Check sheet for the modelled part. Datum: model origin and axes. Units: mm. A direction names the side the tool comes from. Round coordinates to 2 decimals unless told otherwise and drop trailing zeros. Write each loop counter-clockwise with the first axis right and the second up, starting at its lowest first coordinate (ties: lowest second). Pieces come first, ordered by that corner, then holes. Notation, with made-up numbers: (-33.5, 33) -> (0.5, 33) arc R33 ccw to (0.5, 62) -> close; hole circle Ø7 at (8, -16.75). An arc over 180 degrees is marked (long way). One line per item, written item: value.
from build123d import *

# Parameters (mm, degrees)
SKETCH_1_R          = 3.9
SKETCH_1_R_2        = 2.2
SKETCH_1_R_3        = 1
EXTRUDE_1_DEPTH     = 0.8
SKETCH_1_4_R        = 2.2
SKETCH_1_4_R_2      = 1
EXTRUDE_2_DEPTH     = 3.2
FILLET_1_R          = 0.2
SKETCH_2_R          = 1.15
CUT_EXTRUDE_1_DEPTH = 0.5
CUT_EXTRUDE_2_REACH = 8.813


with BuildPart() as part:
    # Sketch 1 → Extrude 1 (new body)
    with BuildSketch(Plane.XY):
        Circle(SKETCH_1_R)
        Circle(SKETCH_1_R_2, mode=Mode.SUBTRACT)
        Circle(SKETCH_1_R_2)
        Circle(SKETCH_1_R_3, mode=Mode.SUBTRACT)
    extrude(amount=-EXTRUDE_1_DEPTH)

    # Sketch 1_4 → Extrude 2 (add)
    with BuildSketch(Plane.XY):
        Circle(SKETCH_1_4_R)
        Circle(SKETCH_1_4_R_2, mode=Mode.SUBTRACT)
    extrude(amount=EXTRUDE_2_DEPTH)

    # Fillet 1
    fillet_1_edges = [part.edges().sort_by_distance(p)[0] for p in [
        (-2.2, 0, 3.2),
    ]]
    fillet(fillet_1_edges, radius=FILLET_1_R)

    # Sketch 2 → Cut-Extrude 1 (cut)
    with BuildSketch(Plane(origin=(0, 0, -0.8), x_dir=(-1, 0, 0), z_dir=(0, 0, -1))):
        Circle(SKETCH_2_R)
    extrude(amount=-CUT_EXTRUDE_1_DEPTH, mode=Mode.SUBTRACT)

    # Sketch 3 → Cut-Extrude 2 (cut, up to next)
    with BuildSketch(Plane(origin=(0, 0, -0.8), x_dir=(-1, 0, 0), z_dir=(0, 0, -1)), mode=Mode.PRIVATE) as cut_extrude_2_sk1:
        with BuildLine():
            Line((-0.7, -2.085665361), (-0.7, -2.711088342))
            ThreePointArc((-0.7, -2.711088342), (0, -2.8), (0.7, -2.711088342))
            Line((0.7, -2.711088342), (0.7, -2.085665361))
            ThreePointArc((0.7, -2.085665361), (0, -2.2), (-0.7, -2.085665361))
        make_face()
    cut_extrude_2_tool1 = extrude(cut_extrude_2_sk1.sketch, amount=-CUT_EXTRUDE_2_REACH, mode=Mode.PRIVATE) & part.part
    # Sketch 3 → Cut-Extrude 2 (cut, up to next)
    with BuildSketch(Plane(origin=(0, 0, -0.8), x_dir=(-1, 0, 0), z_dir=(0, 0, -1)), mode=Mode.PRIVATE) as cut_extrude_2_sk2:
        with BuildLine():
            ThreePointArc((0.7, 2.711088342), (0, 2.8), (-0.7, 2.711088342))
            Line((-0.7, 2.711088342), (-0.7, 2.085665361))
            ThreePointArc((-0.7, 2.085665361), (0, 2.2), (0.7, 2.085665361))
            Line((0.7, 2.085665361), (0.7, 2.711088342))
        make_face()
    cut_extrude_2_tool2 = extrude(cut_extrude_2_sk2.sketch, amount=-CUT_EXTRUDE_2_REACH, mode=Mode.PRIVATE) & part.part
    # Sketch 3 → Cut-Extrude 2 (cut, up to next)
    with BuildSketch(Plane(origin=(0, 0, -0.8), x_dir=(-1, 0, 0), z_dir=(0, 0, -1)), mode=Mode.PRIVATE) as cut_extrude_2_sk3:
        with BuildLine():
            Line((-0.7, -2.085665361), (-0.7, -2.711088342))
            ThreePointArc((-0.7, -2.711088342), (0, -2.8), (0.7, -2.711088342))
            Line((0.7, -2.711088342), (0.7, -2.085665361))
            ThreePointArc((0.7, -2.085665361), (0, -2.2), (-0.7, -2.085665361))
        make_face()
    cut_extrude_2_tool3 = extrude(cut_extrude_2_sk3.sketch, amount=-CUT_EXTRUDE_2_REACH, mode=Mode.PRIVATE) & part.part
    # Sketch 3 → Cut-Extrude 2 (cut, up to next)
    with BuildSketch(Plane(origin=(0, 0, -0.8), x_dir=(-1, 0, 0), z_dir=(0, 0, -1)), mode=Mode.PRIVATE) as cut_extrude_2_sk4:
        with BuildLine():
            ThreePointArc((0.7, 2.711088342), (0, 2.8), (-0.7, 2.711088342))
            Line((-0.7, 2.711088342), (-0.7, 2.085665361))
            ThreePointArc((-0.7, 2.085665361), (0, 2.2), (0.7, 2.085665361))
            Line((0.7, 2.085665361), (0.7, 2.711088342))
        make_face()
    cut_extrude_2_tool4 = extrude(cut_extrude_2_sk4.sketch, amount=-CUT_EXTRUDE_2_REACH, mode=Mode.PRIVATE) & part.part
    # Sketch 3 → Cut-Extrude 2 (cut, up to next)
    with BuildSketch(Plane(origin=(0, 0, -0.8), x_dir=(-1, 0, 0), z_dir=(0, 0, -1)), mode=Mode.PRIVATE) as cut_extrude_2_sk5:
        with BuildLine():
            ThreePointArc((-2.711088342, 0.7), (-2.8, 0), (-2.711088342, -0.7))
            Line((-2.711088342, -0.7), (-2.085665361, -0.7))
            ThreePointArc((-2.085665361, -0.7), (-2.2, 0), (-2.085665361, 0.7))
            Line((-2.085665361, 0.7), (-2.711088342, 0.7))
        make_face()
    cut_extrude_2_tool5 = extrude(cut_extrude_2_sk5.sketch, amount=-CUT_EXTRUDE_2_REACH, mode=Mode.PRIVATE) & part.part
    # Sketch 3 → Cut-Extrude 2 (cut, up to next)
    with BuildSketch(Plane(origin=(0, 0, -0.8), x_dir=(-1, 0, 0), z_dir=(0, 0, -1)), mode=Mode.PRIVATE) as cut_extrude_2_sk6:
        with BuildLine():
            Line((2.085665361, -0.7), (2.711088342, -0.7))
            ThreePointArc((2.711088342, -0.7), (2.77768315, -0.352812019), (2.8, 0))
            ThreePointArc((2.8, 0), (2.77768315, 0.352812019), (2.711088342, 0.7))
            Line((2.711088342, 0.7), (2.085665361, 0.7))
            ThreePointArc((2.085665361, 0.7), (2.1712282, 0.354637988), (2.2, 0))
            ThreePointArc((2.2, 0), (2.1712282, -0.354637988), (2.085665361, -0.7))
        make_face()
    cut_extrude_2_tool6 = extrude(cut_extrude_2_sk6.sketch, amount=-CUT_EXTRUDE_2_REACH, mode=Mode.PRIVATE) & part.part
    # Sketch 3 → Cut-Extrude 2 (cut, up to next)
    with BuildSketch(Plane(origin=(0, 0, -0.8), x_dir=(-1, 0, 0), z_dir=(0, 0, -1)), mode=Mode.PRIVATE) as cut_extrude_2_sk7:
        with BuildLine():
            ThreePointArc((-2.711088342, 0.7), (-2.8, 0), (-2.711088342, -0.7))
            Line((-2.711088342, -0.7), (-2.085665361, -0.7))
            ThreePointArc((-2.085665361, -0.7), (-2.2, 0), (-2.085665361, 0.7))
            Line((-2.085665361, 0.7), (-2.711088342, 0.7))
        make_face()
    cut_extrude_2_tool7 = extrude(cut_extrude_2_sk7.sketch, amount=-CUT_EXTRUDE_2_REACH, mode=Mode.PRIVATE) & part.part
    # Sketch 3 → Cut-Extrude 2 (cut, up to next)
    with BuildSketch(Plane(origin=(0, 0, -0.8), x_dir=(-1, 0, 0), z_dir=(0, 0, -1)), mode=Mode.PRIVATE) as cut_extrude_2_sk8:
        with BuildLine():
            Line((2.085665361, -0.7), (2.711088342, -0.7))
            ThreePointArc((2.711088342, -0.7), (2.77768315, -0.352812019), (2.8, 0))
            ThreePointArc((2.8, 0), (2.77768315, 0.352812019), (2.711088342, 0.7))
            Line((2.711088342, 0.7), (2.085665361, 0.7))
            ThreePointArc((2.085665361, 0.7), (2.1712282, 0.354637988), (2.2, 0))
            ThreePointArc((2.2, 0), (2.1712282, -0.354637988), (2.085665361, -0.7))
        make_face()
    cut_extrude_2_tool8 = extrude(cut_extrude_2_sk8.sketch, amount=-CUT_EXTRUDE_2_REACH, mode=Mode.PRIVATE) & part.part
    add(cut_extrude_2_tool1.solids().sort_by_distance((0, -2.466051, -0.8))[0], mode=Mode.SUBTRACT)
    add(cut_extrude_2_tool2.solids().sort_by_distance((0, 2.466051, -0.8))[0], mode=Mode.SUBTRACT)
    add(cut_extrude_2_tool3.solids().sort_by_distance((0, -2.466051, -0.8))[0], mode=Mode.SUBTRACT)
    add(cut_extrude_2_tool4.solids().sort_by_distance((0, 2.466051, -0.8))[0], mode=Mode.SUBTRACT)
    add(cut_extrude_2_tool5.solids().sort_by_distance((2.466051, 0, -0.8))[0], mode=Mode.SUBTRACT)
    add(cut_extrude_2_tool6.solids().sort_by_distance((-2.466051, 0, -0.8))[0], mode=Mode.SUBTRACT)
    add(cut_extrude_2_tool7.solids().sort_by_distance((2.466051, 0, -0.8))[0], mode=Mode.SUBTRACT)
    add(cut_extrude_2_tool8.solids().sort_by_distance((-2.466051, 0, -0.8))[0], mode=Mode.SUBTRACT)


solid = part.part
Item 1: Sectioned sample at A-A on x = 0. Enter the section's corners in (y, z), and give its area (3 significant figures).
Answer:
outline: (-3.9, -0.8) -> (-2.8, -0.8) -> (-2.8, 0) -> (-3.9, 0) -> close; (-2.2, -0.8) -> (-1.15, -0.8) -> (-1.15, -0.3) -> (-1, -0.3) -> (-1, 3.2) -> (-2, 3.2) arc R0.2 ccw to (-2.2, 3) -> close; (1, -0.3) -> (1.15, -0.3) -> (1.15, -0.8) -> (2.2, -0.8) -> (2.2, 3) arc R0.2 ccw to (2, 3.2) -> (1, 3.2) -> close; (2.8, -0.8) -> (3.9, -0.8) -> (3.9, 0) -> (2.8, 0) -> close
area: 11.2 mm^2
Item 2: Depth check by flat-ended pin: P1, Ø0.5, axis at y = 2, z = -0.5, coming from the -X side; P2, Ø0.5, axis at x = -2.5, z = -0.5, coming from the +Y side; P3, Ø0.5, axis at x = -2.5, z = -0.5, coming from the -Y side. Enter the tip coordinate at first touch or a pass-through.
Answer:
P1: stops at x = -3.49
P2: stops at y = 3.19
P3: stops at y = -3.19
Item 3: Sectioned sample at B-B on z = -0.1. Enter the section's corners in (x, y).
Answer:
outline: circle Ø7.8 at (0, 0); hole (-2.71, -0.7) -> (-2.09, -0.7) arc R2.2 cw to (-2.09, 0.7) -> (-2.71, 0.7) arc R2.8 ccw to start; hole circle Ø2 at (0, 0); hole (-0.7, -2.71) arc R2.8 ccw to (0.7, -2.71) -> (0.7, -2.09) arc R2.2 cw to (-0.7, -2.09) -> close; hole (-0.7, 2.09) arc R2.2 cw to (0.7, 2.09) -> (0.7, 2.71) arc R2.8 ccw to (-0.7, 2.71) -> close; hole (2.09, -0.7) -> (2.71, -0.7) arc R2.8 ccw to (2.71, 0.7) -> (2.09, 0.7) arc R2.2 cw to start
Item 4: Tool access check on faces 4 (the cylindrical face through (0.91, -0.7, -0.55)), 5 (the flat face through (1, -1, 3.2)), 6 (the flat face through (2, -2, 0)). Record the directions out of +Z, -Z, +X, -X, +Y, -Y that give a thin tool (end or side, any length) a straight path to the whole face; none if there is none.
Answer:
face 4: -Z
face 5: +Z, +X, -X, +Y, -Y
face 6: +Z
Item 5: Mould release check, pull along X, two halves, no side actions. Record for faces 1 (the cylindrical face through (-2.87, 2.64, -0.39)), 2 (the cylindrical face through (0, -1, 1)), 3 (the flat face through (-1, -1, -0.8)): pulls with the +X half, pulls with the -X half, needs draft (parallel to the pull), parting line crosses it, or undercut.
Answer:
face 1: parting line crosses it
face 2: undercut
face 3: needs draft
Item 6: Thickness scan on line 1 (Y direction, x = 0, z = -0.5); line 2 (Y direction, x = 0, z = 2); line 3 (Z direction, x = 3.25, y = 0). Record the ranges inside material, lowest first.
Answer:
line 1: y = -3.9 to -2.8, -2.2 to -1.15, 1.15 to 2.2, 2.8 to 3.9
line 2: y = -2.2 to -1, 1 to 2.2
line 3: z = -0.8 to 0
Item 7: Sectioned sample at C-C on z = 1.25. Enter the section's corners in (x, y).
Answer:
outline: circle Ø4.4 at (0, 0); hole circle Ø2 at (0, 0)
